```python
from build123d import *

# Parameters (mm, degrees)
EXTRUDE_1_DEPTH     = 270
SHELL_6_T           = -3
SKETCH_8_W          = 45
SKETCH_8_H          = 45
CUT_EXTRUDE_1_DEPTH = 85.852813742
SKETCH_8_5_R        = 1.75
SKETCH_8_5_W        = 45
SKETCH_8_5_H        = 45
SKETCH_8_5_W_2      = 37
SKETCH_8_5_H_2      = 22
CUT_EXTRUDE_3_DEPTH = 10
SKETCH_10_R         = 3
CUT_EXTRUDE_4_DEPTH = 3
SKETCH_15_R         = 1.5
CUT_EXTRUDE_5_DEPTH = 3


with BuildPart() as part:
    # Sketch 1 → Extrude 1 (new body)
    with BuildSketch(Plane.XY):
        Polygon((-93.609952443, -20), (6.390047557, -20), (6.390047557, 0), (-8.609952443, 0), (-8.609952443, 15), (-83.609952443, 90), (-93.609952443, 90), align=None)
    extrude(amount=EXTRUDE_1_DEPTH)

    # Shell 6
    shell_6_openings = [part.faces().sort_by_distance(p)[0] for p in [
        (-93.609952443, 35, 135),
    ]]
    offset(amount=SHELL_6_T, openings=shell_6_openings, kind=Kind.INTERSECTION)

    # Sketch 8 → Cut-Extrude 1 (cut, through all)
    with BuildSketch(Plane(origin=(3.195023779, 3.195023779, 0), x_dir=(0, 0, -1), z_dir=(0.707106781, 0.707106781, 0))):
        with Locations((-237.5, 92.760774654)):
            Rectangle(SKETCH_8_W, SKETCH_8_H)
    extrude(amount=-CUT_EXTRUDE_1_DEPTH, mode=Mode.SUBTRACT)

    # Sketch 8_5 → Cut-Extrude 3 (cut)
    with BuildSketch(Plane(origin=(3.195023779, 3.195023779, 0), x_dir=(0, 0, -1), z_dir=(0.707106781, 0.707106781, 0))):
        with Locations((-19.5, 45.760774654)):
            Circle(SKETCH_8_5_R)
        with Locations((-15.5, 45.760774654)):
            Circle(SKETCH_8_5_R)
        with Locations((-9.5, 45.760774654)):
            Circle(SKETCH_8_5_R)
        with Locations((-5.5, 45.760774654)):
            Circle(SKETCH_8_5_R)
        with Locations((-27.5, 45.760774654)):
            Circle(SKETCH_8_5_R)
        with Locations((-31.5, 45.760774654)):
            Circle(SKETCH_8_5_R)
        with Locations((-37.5, 45.760774654)):
            Circle(SKETCH_8_5_R)
        with Locations((-41.5, 45.760774654)):
            Circle(SKETCH_8_5_R)
        with Locations((-5.5, 35.760774654)):
            Circle(SKETCH_8_5_R)
        with Locations((-9.5, 35.760774654)):
            Circle(SKETCH_8_5_R)
        with Locations((-15.5, 35.760774654)):
            Circle(SKETCH_8_5_R)
        with Locations((-19.5, 35.760774654)):
            Circle(SKETCH_8_5_R)
        with Locations((-27.5, 35.760774654)):
            Circle(SKETCH_8_5_R)
        with Locations((-31.5, 35.760774654)):
            Circle(SKETCH_8_5_R)
        with Locations((-37.5, 35.760774654)):
            Circle(SKETCH_8_5_R)
        with Locations((-41.5, 35.760774654)):
            Circle(SKETCH_8_5_R)
        with Locations((-41.5, 25.760774654)):
            Circle(SKETCH_8_5_R)
        with Locations((-37.5, 25.760774654)):
            Circle(SKETCH_8_5_R)
        with Locations((-31.5, 25.760774654)):
            Circle(SKETCH_8_5_R)
        with Locations((-27.5, 25.760774654)):
            Circle(SKETCH_8_5_R)
        with Locations((-19.5, 25.760774654)):
            Circle(SKETCH_8_5_R)
        with Locations((-15.5, 25.760774654)):
            Circle(SKETCH_8_5_R)
        with Locations((-9.5, 25.760774654)):
            Circle(SKETCH_8_5_R)
        with Locations((-5.5, 25.760774654)):
            Circle(SKETCH_8_5_R)
        with Locations((-19.5, 60.760774654)):
            Circle(SKETCH_8_5_R)
        with Locations((-27.5, 60.760774654)):
            Circle(SKETCH_8_5_R)
        with Locations((-237.5, 41.694757476)):
            Rectangle(SKETCH_8_5_W, SKETCH_8_5_H)
        with Locations((-237.5, 92.760774654)):
            Rectangle(SKETCH_8_5_W, SKETCH_8_5_H)
        with Locations((-182.5, 92.760774654)):
            Rectangle(SKETCH_8_5_W, SKETCH_8_5_H)
        with Locations((-127.5, 92.760774654)):
            Rectangle(SKETCH_8_5_W, SKETCH_8_5_H)
        with Locations((-182.5, 41.694757476)):
            Rectangle(SKETCH_8_5_W, SKETCH_8_5_H)
        with Locations((-72.5, 92.760774654)):
            Rectangle(SKETCH_8_5_W, SKETCH_8_5_H)
        with Locations((-127.5, 41.694757476)):
            Rectangle(SKETCH_8_5_W, SKETCH_8_5_H)
        with Locations((-72.5, 41.694757476)):
            Rectangle(SKETCH_8_5_W, SKETCH_8_5_H)
        with Locations((-23.5, 96.760774654)):
            Rectangle(SKETCH_8_5_W_2, SKETCH_8_5_H_2)
    extrude(amount=-CUT_EXTRUDE_3_DEPTH, mode=Mode.SUBTRACT)

    # Sketch 10 → Cut-Extrude 4 (cut)
    with BuildSketch(Plane(origin=(-8.609952443, 0, 0), x_dir=(0, 0, -1), z_dir=(1, 0, 0))):
        with Locations((-247.5, 7.5)):
            Circle(SKETCH_10_R)
        with Locations((-222.5, 7.5)):
            Circle(SKETCH_10_R)
        with Locations((-97.5, 7.5)):
            Circle(SKETCH_10_R)
        with Locations((-122.5, 7.5)):
            Circle(SKETCH_10_R)
        with Locations((-147.5, 7.5)):
            Circle(SKETCH_10_R)
        with Locations((-172.5, 7.5)):
            Circle(SKETCH_10_R)
        with Locations((-197.5, 7.5)):
            Circle(SKETCH_10_R)
        with Locations((-72.5, 7.5)):
            Circle(SKETCH_10_R)
        with Locations((-47.5, 7.5)):
            Circle(SKETCH_10_R)
        with Locations((-22.5, 7.5)):
            Circle(SKETCH_10_R)
    extrude(amount=-CUT_EXTRUDE_4_DEPTH, mode=Mode.SUBTRACT)

    # Sketch 15 → Cut-Extrude 5 (cut)
    with BuildSketch(Plane.XZ.offset(20)):
        with Locations((-31.109952443, 192.5)):
            Circle(SKETCH_15_R)
        with Locations((-13.609952443, 192.5)):
            Circle(SKETCH_15_R)
        with Locations((-3.609952443, 240)):
            Circle(SKETCH_15_R)
        with Locations((-31.109952443, 240)):
            Circle(SKETCH_15_R)
    extrude(amount=-CUT_EXTRUDE_5_DEPTH, mode=Mode.SUBTRACT)


solid = part.part
```
Geometry check sheet. Reference: the model listing, model coordinates, mm. A direction names the side the tool comes from. Give positions to 0.01 mm unless a question says otherwise; leave off trailing zeros. Order: outer loops, then holes, each group sorted by start corner. A loop starts at its lowest first (then second) coordinate and runs counter-clockwise, first axis right, second up. Notation, with made-up numbers: (34.25, -12) - (88.25, -12) arc R22 cw to (88.25, 24) - close; hole circle Ø2 at (69.25, 76). An arc over 180 degrees is marked (long way). Answer in a Markdown table with one row per item. Add a question column.
Q1. Cross-section at A-A, the plane z = 97.5. Enter the section's corners in (x, y), then the cut area to 3 significant figures.
Q2. Tool access check on faces 1 (the flat face through (-57, 24, 267)), 2 (the cylindrical face through (-10.1, 7.6, 25.5)), 3 (the flat face through (-8.61, 7, 133)). Record the directions out of +Z, -Z, +X, -X, +Y, -Y that give a thin tool (end or side, any length) a straight path to the whole face; none if there is none.
Q3. Material ranges on probe 1 along Z at (x, y) = (-74, 8); probe 2 along Y at (x, z) = (-9.7, 22.5); probe 3 along Y at (x, z) = (-10, 72), recorded low to high. Write a range as from..to.
Q4. Cross-section at D-D, the plane x = -65.5. Enter the section's corners in (y, z), then the cut area to 3 significant figures.
Q5. Cross-section at B-B, the plane z = 222.5. Enter the section's corners in (x, y), then the cut area to 3 significant figures.
Q6. Gauge pin test, flat ends, axial feed: pin 1 (13.5 mm diameter, centred on y = 3.5, z = 152.5, fed in from -X); pin 2 (8 mm diameter, centred on y = 17.5, z = 187, fed in from +X); pin 3 (8 mm diameter, centred on y = 58.5, z = 210.5, fed in from -X). Record the tip position at first contact, or that the pin passes through.
Q7. Mould release check, pull along Z, two halves, no side actions. Record for faces 4 (the flat face through (-55, 24, 0)), 5 (the flat face through (6.39, -10, 133)), 6 (the flat face through (-63, 68, 150)): pulls with the +Z half, pulls with the -Z half, needs draft (parallel to the pull), parting line crosses it, or undercut.
Q8. Cross-section at C-C, the plane y = -11.5. Enter the section's corners in (x, z), then the cut area to 3 significant figures.
Check values:
| question | item | result |
|---|---|---|
| 1 | outline | (-93.61, -20) - (6.39, -20) - (6.39, 0) - (-8.61, 0) - (-8.61, 4.5) - (-11.61, 4.5) - (-11.61, -3) - (3.39, -3) - (3.39, -17) - (-93.61, -17) - close; (-93.61, 87) - (-84.85, 87) - (-11.61, 13.76) - (-11.61, 10.5) - (-8.61, 10.5) - (-8.61, 15) - (-83.61, 90) - (-93.61, 90) - close |
| 1 | area | 764 mm^2 |
| 2 | face 1 | -X |
| 2 | face 2 | +X, -X |
| 2 | face 3 | +Z, -Z, +X, +Y |
| 3 | probe 1 | z = 0..3, 267..270 |
| 3 | probe 2 | y = -20..-17, -3..4.5, 10.5..16.09 |
| 3 | probe 3 | y = -20..-17, -3..4.54, 10.46..16.39 |
| 4 | outline | (-20, 0) - (71.89, 0) - (71.89, 5) - (67.65, 5) - (67.65, 3) - (-17, 3) - (-17, 267) - (67.65, 267) - (67.65, 260) - (71.89, 260) - (71.89, 270) - (-20, 270) - close; (67.65, 42) - (71.89, 42) - (71.89, 50) - (67.65, 50) - close; (67.65, 95) - (71.89, 95) - (71.89, 105) - (67.65, 105) - close; (67.65, 150) - (71.89, 150) - (71.89, 160) - (67.65, 160) - close; (67.65, 205) - (71.89, 205) - (71.89, 215) - (67.65, 215) - close |
| 4 | area | 1,540 mm^2 |
| 5 | outline | (-93.61, -20) - (6.39, -20) - (6.39, 0) - (-8.61, 0) - (-8.61, 4.5) - (-11.61, 4.5) - (-11.61, -3) - (3.39, -3) - (3.39, -17) - (-93.61, -17) - close; (-93.61, 87) - (-84.85, 87) - (-80.43, 82.58) - (-78.31, 84.7) - (-83.61, 90) - (-93.61, 90) - close; (-48.61, 50.76) - (-44.32, 46.47) - (-42.2, 48.59) - (-46.49, 52.88) - close; (-12.5, 14.65) - (-11.61, 13.76) - (-11.61, 10.5) - (-8.61, 10.5) - (-8.61, 15) - (-10.38, 16.77) - close |
| 5 | area | 494 mm^2 |
| 6 | pin 1 | stops at x = -11.61 |
| 6 | pin 2 | stops at x = -8.61 |
| 6 | pin 3 | stops at x = -60.35 |
| 7 | face 4 | pulls with the -Z half |
| 7 | face 5 | needs draft |
| 7 | face 6 | undercut |
| 8 | outline | (-93.61, 0) - (6.39, 0) - (6.39, 270) - (-93.61, 270) - (-93.61, 267) - (3.39, 267) - (3.39, 3) - (-93.61, 3) - close |
| 8 | area | 1,390 mm^2 |
